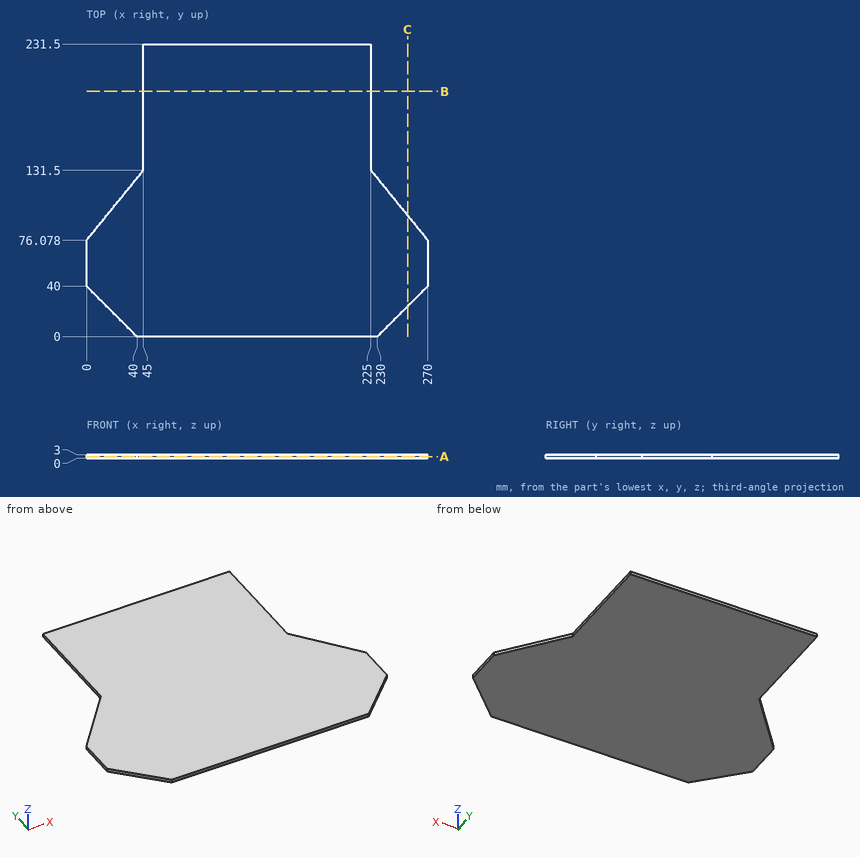
Geometry: see drawing. Coordinates: mm, zero at the bounding-box minimum. Round coordinates to 2 decimals unless told otherwise and drop trailing zeros. Write each loop counter-clockwise with the first axis right and the second up, starting at its lowest first coordinate (ties: lowest second). Pieces come first, ordered by that corner, then holes.
1) Cut plane C-C (x = 254). Return the cut outline in (y, z).
2) Ray query, L1, parallel to X at y = 194.5, z = 1.5; L2, parallel to Y at x = 226.5, z = 0.45; L3, parallel to X at y = 17, z = 1.9. Return the intervals inside material, ascending.
3) Cut plane B-B (y = 194). Return the cut outline in (x, z), then the cut area to 3 significant figures.
4) Cut plane A-A (z = 1.5). Return the cut outline in (x, y), then the cut area to 3 significant figures.
5) Contact query for flat-ended pins moving along their axis: P1, Ø1, axis at x = 37.5, z = 2, coming from the -Y side; P2, Ø1.5, axis at y = 184, z = 1.5, coming from the -X side. Output: stop coordinate, or through.
Geometry says:
1. outline: (24, 0) - (95.78, 0) - (95.78, 3) - (24, 3) - close
2. L1: x = 45 to 225
2. L2: y = 0 to 129.65
2. L3: x = 23 to 247
3. outline: (45, 0) - (225, 0) - (225, 3) - (45, 3) - close
3. area: 540 mm2
4. outline: (0, 40) - (40, 0) - (230, 0) - (270, 40) - (270, 76.08) - (225, 131.5) - (225, 231.5) - (45, 231.5) - (45, 131.5) - (0, 76.08) - close
4. area: 49,400 mm2
5. P1: stops at y = 2
5. P2: stops at x = 45
